```python
from build123d import *

# Parameters (mm, degrees)
SKETCH1_W                 = 65.925
SKETCH1_H                 = 70
BOSS_EXTRUDE1_DEPTH       = 1.5
CUT_EXTRUDE1_REACH        = 137.268
SKETCH4_W                 = 8
SKETCH4_H                 = 4.5
SKETCH4_W_2               = 5
SKETCH4_H_2               = 1.5
BOSS_EXTRUDE2_DEPTH       = 3
MIRROR2_COPY_1_SKETCH_W   = 8
MIRROR2_COPY_1_SKETCH_H   = 4.5
MIRROR2_COPY_1_SKETCH_W_2 = 5
MIRROR2_COPY_1_SKETCH_H_2 = 1.5
MIRROR2_COPY_1_DEPTH      = 3


with BuildPart() as part:
    # Sketch1 → Boss-Extrude1 (new body)
    with BuildSketch(Plane.XY):
        with Locations((88.1375, 25.25)):
            Rectangle(SKETCH1_W, SKETCH1_H)
    extrude(amount=BOSS_EXTRUDE1_DEPTH)

    # Sketch2 → Cut-Extrude1 (cut, up to next)
    with BuildSketch(Plane.XY.offset(1.5), mode=Mode.PRIVATE) as cut_extrude1_sk1:
        with BuildLine():
            Line((92.897490926, 22.3), (92.9875, 22.3))
            ThreePointArc((92.9875, 22.3), (95.9375, 25.25), (92.9875, 28.2))
            Line((92.9875, 28.2), (92.897490926, 28.2))
            ThreePointArc((92.897490926, 28.2), (81.1375, 25.25), (92.897490926, 22.3))
        make_face()
    cut_extrude1_tool1 = extrude(cut_extrude1_sk1.sketch, amount=-CUT_EXTRUDE1_REACH, mode=Mode.PRIVATE) & part.part
    add(cut_extrude1_tool1.solids().sort_by_distance((87.980915, 25.25, 1.5))[0], mode=Mode.SUBTRACT)

    # Sketch4 → Boss-Extrude2 (add)
    with BuildSketch(Plane(origin=(0, 0, 0), x_dir=(-1, 0, 0), z_dir=(0, 0, -1))):
        with Locations((-115.6, 56.5)):
            Rectangle(SKETCH4_W, SKETCH4_H)
        with Locations((-115.6, 56.5)):
            Rectangle(SKETCH4_W_2, SKETCH4_H_2, mode=Mode.SUBTRACT)
    boss_extrude2 = extrude(amount=BOSS_EXTRUDE2_DEPTH)

    # Mirror1: Boss-Extrude2 across plane
    add(boss_extrude2.mirror(Plane(origin=(88.1375, 0, 0), x_dir=(0, 0, 1), z_dir=(1, 0, 0))))

    # Mirror2: Boss-Extrude2 across plane
    add(boss_extrude2.mirror(Plane.ZX.offset(25.25)))

    # Mirror2 copy 1 sketch → Mirror2 copy 1 (add)
    with BuildSketch(Plane(origin=(176.275, 50.5, 0), x_dir=(1, 0, 0), z_dir=(0, 0, -1))):
        with Locations((-115.6, 56.5)):
            Rectangle(MIRROR2_COPY_1_SKETCH_W, MIRROR2_COPY_1_SKETCH_H)
        with Locations((-115.6, 56.5)):
            Rectangle(MIRROR2_COPY_1_SKETCH_W_2, MIRROR2_COPY_1_SKETCH_H_2, mode=Mode.SUBTRACT)
    extrude(amount=MIRROR2_COPY_1_DEPTH)


solid = part.part
```
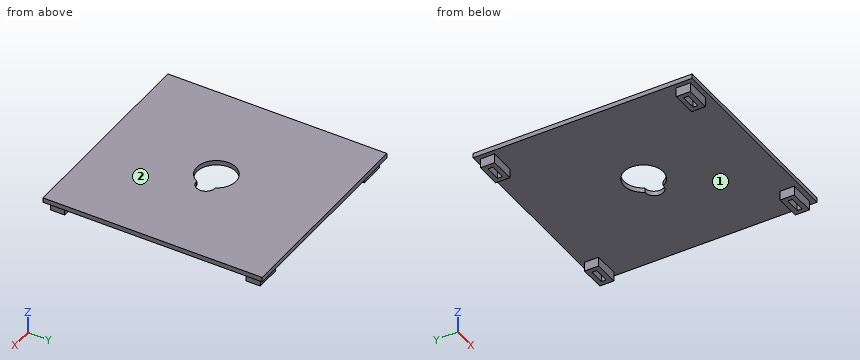
For this review, take the finished solid that the model builds, in its own axes (mm). Face numbers are marked on the shaded views. Coordinates: 2 decimals unless noted, no trailing zeros. Order: outer loops, then holes, each group sorted by start corner. A loop starts at its lowest first (then second) coordinate and runs counter-clockwise, first axis right, second up. Notation, with made-up numbers: (-25.5, 80) -> (6.5, 80) arc R17 ccw to (6.5, 102) -> close; hole circle Ø5 at (37, 43). An arc over 180 degrees is marked (long way). Use CSV: the item, a comma, the result in double quotes. Start each with the question number.
Item 1: Draft analysis for pull direction Y (two halves, no side actions). For the marked faces 1 and 2, state which applies: pulls with the +Y half, pulls with the -Y half, needs draft (parallel to the pull), parting line crosses it, or undercut.
Item 2: Wall thickness on probe 1 along Y at (x, z) = (116.5, -0.25); probe 2 along X at (y, z) = (25.25, 0.9) (1 decimal); probe 3 along X at (y, z) = (-4.5, -2.3) (3 decimals): over which ranges is each line inside the solid? List them lowest first.
Item 3: Insertion check: pin 1 (0.9 mm diameter, centred on y = -5, z = -1.5, fed in from -X) (3 decimals); pin 2 (1.5 mm diameter, centred on x = 62, z = -1.5, fed in from +Y); pin 3 (1.2 mm diameter, centred on x = 115.5, y = -6, fed in from -Z); pin 4 (1.6 mm diameter, centred on x = 60, y = -6, fed in from -Z). Each pin has a flat end and moves straight along its axis. Give the tip position at first contact, or say it passes through.
Item 4: We need section A-A, the plane z = -1.8. Give the number of separate pieces and of enclosed holes in the cut face, then the cut area to 3 significant figures.
Item 5: We need section B-B, the plane y = 25.25. Give the boundary of the cut face in (x, z) (1 decimal).
Item 6: We need section D-D, the plane y = -0.5. Give the boundary of the cut face in (x, z) (3 decimals), then the cut area to 3 significant figures.
Item 7: We need section C-C, the plane x = 87. Give the boundary of the cut face in (y, z), then the cut area to 3 significant figures.
Derived:
1,face 1,"undercut"
1,face 2,"needs draft"
2,probe 1,"y = -8.25 to -6.75, -5.25 to -3.75, 54.25 to 55.75, 57.25 to 58.75"
2,probe 2,"x = 55.2 to 81.1, 95.9 to 121.1"
2,probe 3,"x = 56.675 to 64.675, 111.6 to 119.6"
3,pin 1,"stops at x = 56.675"
3,pin 2,"stops at y = 58.75"
3,pin 3,"stops at z = 0"
3,pin 4,"stops at z = -3"
4,separate pieces,"4"
4,enclosed holes,"4"
4,area,"114 mm^2"
5,outline,"(55.2, 0) -> (81.1, 0) -> (81.1, 1.5) -> (55.2, 1.5) -> close; (95.9, 0) -> (121.1, 0) -> (121.1, 1.5) -> (95.9, 1.5) -> close"
6,outline,"(55.175, 0) -> (121.1, 0) -> (121.1, 1.5) -> (55.175, 1.5) -> close"
6,area,"98.9 mm^2"
7,outline,"(-9.75, 0) -> (19.01, 0) -> (19.01, 1.5) -> (-9.75, 1.5) -> close; (31.49, 0) -> (60.25, 0) -> (60.25, 1.5) -> (31.49, 1.5) -> close"
7,area,"86.3 mm^2"
